```python
from build123d import *

# Parameters (mm, degrees)
BOSS_EXTRUDE1_DEPTH = 200
SKETCH2_R           = 2.5
CUT_EXTRUDE1_DEPTH  = 203.484567313


with BuildPart() as part:
    # Sketch1 → Boss-Extrude1 (new body)
    with BuildSketch(Plane.XY):
        with BuildLine():
            Line((-8.5, 10), (-3.8, 10))
            ThreePointArc((-3.8, 10), (-3.658578644, 9.941421356), (-3.6, 9.8))
            Line((-3.6, 9.8), (-3.6, 9.7))
            ThreePointArc((-3.6, 9.7), (-3.541421356, 9.558578644), (-3.4, 9.5))
            Line((-3.4, 9.5), (-3.3, 9.5))
            ThreePointArc((-3.3, 9.5), (-3.158578644, 9.441421356), (-3.1, 9.3))
            Line((-3.1, 9.3), (3.1, 9.3))
            ThreePointArc((3.1, 9.3), (3.158578644, 9.441421356), (3.3, 9.5))
            Line((3.3, 9.5), (3.4, 9.5))
            ThreePointArc((3.4, 9.5), (3.541421356, 9.558578644), (3.6, 9.7))
            Line((3.6, 9.7), (3.6, 9.8))
            ThreePointArc((3.6, 9.8), (3.658578644, 9.941421356), (3.8, 10))
            Line((3.8, 10), (8.5, 10))
            Line((8.5, 10), (11.5, 10))
            Line((11.5, 10), (16.2, 10))
            ThreePointArc((16.2, 10), (16.341421356, 9.941421356), (16.4, 9.8))
            Line((16.4, 9.8), (16.4, 9.7))
            ThreePointArc((16.4, 9.7), (16.458578644, 9.558578644), (16.6, 9.5))
            Line((16.6, 9.5), (16.7, 9.5))
            ThreePointArc((16.7, 9.5), (16.841421356, 9.441421356), (16.9, 9.3))
            Line((16.9, 9.3), (16.9, 8.2))
            Line((16.9, 8.2), (14.7, 8.2))
            ThreePointArc((14.7, 8.2), (14.558578644, 8.141421356), (14.5, 8))
            Line((14.5, 8), (14.5, 6.560660172))
            Line((14.5, 6.560660172), (17.102081528, 3.958578644))
            ThreePointArc((17.102081528, 3.958578644), (17.166966198, 3.915224093), (17.243502884, 3.9))
            Line((17.243502884, 3.9), (22.756497116, 3.9))
            ThreePointArc((22.756497116, 3.9), (22.833033802, 3.915224093), (22.897918472, 3.958578644))
            Line((22.897918472, 3.958578644), (25.5, 6.560660172))
            Line((25.5, 6.560660172), (25.5, 8))
            ThreePointArc((25.5, 8), (25.441421356, 8.141421356), (25.3, 8.2))
            Line((25.3, 8.2), (23.1, 8.2))
            Line((23.1, 8.2), (23.1, 9.3))
            ThreePointArc((23.1, 9.3), (23.158578644, 9.441421356), (23.3, 9.5))
            Line((23.3, 9.5), (23.4, 9.5))
            ThreePointArc((23.4, 9.5), (23.541421356, 9.558578644), (23.6, 9.7))
            Line((23.6, 9.7), (23.6, 9.8))
            ThreePointArc((23.6, 9.8), (23.658578644, 9.941421356), (23.8, 10))
            Line((23.8, 10), (28.5, 10))
            ThreePointArc((28.5, 10), (29.560660172, 9.560660172), (30, 8.5))
            Line((30, 8.5), (30, 3.8))
            ThreePointArc((30, 3.8), (29.941421356, 3.658578644), (29.8, 3.6))
            Line((29.8, 3.6), (29.7, 3.6))
            ThreePointArc((29.7, 3.6), (29.558578644, 3.541421356), (29.5, 3.4))
            Line((29.5, 3.4), (29.5, 3.3))
            ThreePointArc((29.5, 3.3), (29.441421356, 3.158578644), (29.3, 3.1))
            Line((29.3, 3.1), (28.2, 3.1))
            Line((28.2, 3.1), (28.2, 5.3))
            ThreePointArc((28.2, 5.3), (28.141421356, 5.441421356), (28, 5.5))
            Line((28, 5.5), (26.560660172, 5.5))
            Line((26.560660172, 5.5), (23.958578644, 2.897918472))
            ThreePointArc((23.958578644, 2.897918472), (23.915224093, 2.833033802), (23.9, 2.756497116))
            Line((23.9, 2.756497116), (23.9, -2.756497116))
            ThreePointArc((23.9, -2.756497116), (23.915224093, -2.833033802), (23.958578644, -2.897918472))
            Line((23.958578644, -2.897918472), (26.560660172, -5.5))
            Line((26.560660172, -5.5), (28, -5.5))
            ThreePointArc((28, -5.5), (28.141421356, -5.441421356), (28.2, -5.3))
            Line((28.2, -5.3), (28.2, -3.1))
            Line((28.2, -3.1), (29.3, -3.1))
            ThreePointArc((29.3, -3.1), (29.441421356, -3.158578644), (29.5, -3.3))
            Line((29.5, -3.3), (29.5, -3.4))
            ThreePointArc((29.5, -3.4), (29.558578644, -3.541421356), (29.7, -3.6))
            Line((29.7, -3.6), (29.8, -3.6))
            ThreePointArc((29.8, -3.6), (29.941421356, -3.658578644), (30, -3.8))
            Line((30, -3.8), (30, -8.5))
            ThreePointArc((30, -8.5), (29.560660172, -9.560660172), (28.5, -10))
            Line((28.5, -10), (23.8, -10))
            ThreePointArc((23.8, -10), (23.658578644, -9.941421356), (23.6, -9.8))
            Line((23.6, -9.8), (23.6, -9.7))
            ThreePointArc((23.6, -9.7), (23.541421356, -9.558578644), (23.4, -9.5))
            Line((23.4, -9.5), (23.3, -9.5))
            ThreePointArc((23.3, -9.5), (23.158578644, -9.441421356), (23.1, -9.3))
            Line((23.1, -9.3), (23.1, -8.2))
            Line((23.1, -8.2), (25.3, -8.2))
            ThreePointArc((25.3, -8.2), (25.441421356, -8.141421356), (25.5, -8))
            Line((25.5, -8), (25.5, -6.560660172))
            Line((25.5, -6.560660172), (22.897918472, -3.958578644))
            ThreePointArc((22.897918472, -3.958578644), (22.833033802, -3.915224093), (22.756497116, -3.9))
            Line((22.756497116, -3.9), (17.243502884, -3.9))
            ThreePointArc((17.243502884, -3.9), (17.166966198, -3.915224093), (17.102081528, -3.958578644))
            Line((17.102081528, -3.958578644), (14.5, -6.560660172))
            Line((14.5, -6.560660172), (14.5, -8))
            ThreePointArc((14.5, -8), (14.558578644, -8.141421356), (14.7, -8.2))
            Line((14.7, -8.2), (16.9, -8.2))
            Line((16.9, -8.2), (16.9, -9.3))
            ThreePointArc((16.9, -9.3), (16.841421356, -9.441421356), (16.7, -9.5))
            Line((16.7, -9.5), (16.6, -9.5))
            ThreePointArc((16.6, -9.5), (16.458578644, -9.558578644), (16.4, -9.7))
            Line((16.4, -9.7), (16.4, -9.8))
            ThreePointArc((16.4, -9.8), (16.341421356, -9.941421356), (16.2, -10))
            Line((16.2, -10), (11.5, -10))
            Line((11.5, -10), (8.5, -10))
            Line((8.5, -10), (3.8, -10))
            ThreePointArc((3.8, -10), (3.658578644, -9.941421356), (3.6, -9.8))
            Line((3.6, -9.8), (3.6, -9.7))
            ThreePointArc((3.6, -9.7), (3.541421356, -9.558578644), (3.4, -9.5))
            Line((3.4, -9.5), (3.3, -9.5))
            Line((3.3, -9.5), (-3.3, -9.5))
            Line((-3.3, -9.5), (-3.4, -9.5))
            ThreePointArc((-3.4, -9.5), (-3.541421356, -9.558578644), (-3.6, -9.7))
            Line((-3.6, -9.7), (-3.6, -9.8))
            ThreePointArc((-3.6, -9.8), (-3.658578644, -9.941421356), (-3.8, -10))
            Line((-3.8, -10), (-8.5, -10))
            ThreePointArc((-8.5, -10), (-9.560660172, -9.560660172), (-10, -8.5))
            Line((-10, -8.5), (-10, -3.8))
            ThreePointArc((-10, -3.8), (-9.941421356, -3.658578644), (-9.8, -3.6))
            Line((-9.8, -3.6), (-9.7, -3.6))
            ThreePointArc((-9.7, -3.6), (-9.558578644, -3.541421356), (-9.5, -3.4))
            Line((-9.5, -3.4), (-9.5, -3.3))
            ThreePointArc((-9.5, -3.3), (-9.441421356, -3.158578644), (-9.3, -3.1))
            Line((-9.3, -3.1), (-8.2, -3.1))
            Line((-8.2, -3.1), (-8.2, -5.3))
            ThreePointArc((-8.2, -5.3), (-8.141421356, -5.441421356), (-8, -5.5))
            Line((-8, -5.5), (-6.560660172, -5.5))
            Line((-6.560660172, -5.5), (-3.958578644, -2.897918472))
            ThreePointArc((-3.958578644, -2.897918472), (-3.915224093, -2.833033802), (-3.9, -2.756497116))
            Line((-3.9, -2.756497116), (-3.9, 2.756497116))
            ThreePointArc((-3.9, 2.756497116), (-3.915224093, 2.833033802), (-3.958578644, 2.897918472))
            Line((-3.958578644, 2.897918472), (-6.560660172, 5.5))
            Line((-6.560660172, 5.5), (-8, 5.5))
            ThreePointArc((-8, 5.5), (-8.141421356, 5.441421356), (-8.2, 5.3))
            Line((-8.2, 5.3), (-8.2, 3.1))
            Line((-8.2, 3.1), (-9.3, 3.1))
            ThreePointArc((-9.3, 3.1), (-9.441421356, 3.158578644), (-9.5, 3.3))
            Line((-9.5, 3.3), (-9.5, 3.4))
            ThreePointArc((-9.5, 3.4), (-9.558578644, 3.541421356), (-9.7, 3.6))
            Line((-9.7, 3.6), (-9.8, 3.6))
            ThreePointArc((-9.8, 3.6), (-9.941421356, 3.658578644), (-10, 3.8))
            Line((-10, 3.8), (-10, 8.5))
            ThreePointArc((-10, 8.5), (-9.560660172, 9.560660172), (-8.5, 10))
        make_face()
        with BuildLine():
            Line((3.9, 2.756497116), (3.9, -2.756497116))
            ThreePointArc((3.9, -2.756497116), (3.915224093, -2.833033802), (3.958578644, -2.897918472))
            Line((3.958578644, -2.897918472), (6.560660172, -5.5))
            Line((6.560660172, -5.5), (6.560660172, -8.2))
            Line((6.560660172, -8.2), (13.439339828, -8.2))
            Line((13.439339828, -8.2), (13.439339828, -5.5))
            Line((13.439339828, -5.5), (16.041421356, -2.897918472))
            ThreePointArc((16.041421356, -2.897918472), (16.084775907, -2.833033802), (16.1, -2.756497116))
            Line((16.1, -2.756497116), (16.1, 2.756497116))
            ThreePointArc((16.1, 2.756497116), (16.084775907, 2.833033802), (16.041421356, 2.897918472))
            Line((16.041421356, 2.897918472), (13.439339828, 5.5))
            Line((13.439339828, 5.5), (13.439339828, 8.2))
            Line((13.439339828, 8.2), (6.560660172, 8.2))
            Line((6.560660172, 8.2), (6.560660172, 5.5))
            Line((6.560660172, 5.5), (3.958578644, 2.897918472))
            ThreePointArc((3.958578644, 2.897918472), (3.915224093, 2.833033802), (3.9, 2.756497116))
        make_face(mode=Mode.SUBTRACT)
    extrude(amount=BOSS_EXTRUDE1_DEPTH)

    # Sketch2 → Cut-Extrude1 (cut, through all)
    with BuildSketch(Plane.XY.offset(200)):
        Circle(SKETCH2_R)
        with Locations(Location((20, 0, 0), (0, 0, 180))):
            Circle(SKETCH2_R)
    extrude(amount=-CUT_EXTRUDE1_DEPTH, mode=Mode.SUBTRACT)


solid = part.part
```
Geometry check sheet. Reference: the model listing, model coordinates, mm. A direction names the side the tool comes from. Coordinates: 2 decimals unless noted, no trailing zeros. Order: outer loops, then holes, each group sorted by start corner. A loop starts at its lowest first (then second) coordinate and runs counter-clockwise, first axis right, second up.
Item 1: Scan lines: line 1 along X through (y, z) = (-7.25, 171); line 2 along Y through (x, z) = (0, 93); line 3 along X through (y, z) = (2.25, 39.5). Record each from-to range of solid material in increasing order.
Item 2: Mould release check, pull along Y, two halves, no side actions. Record for faces 4 (the flat face through (10, 10, 99)), 5 (the flat face through (10, -8.2, 99)), 6 (the flat face through (6, 7, 200)): released by +Y, released by -Y, zero draft, split by the parting line, or undercut.
Item 3: Section check A-A (y = 0). Enter the section's corners in (x, z).
Item 4: Tool access check on faces 1 (the flat face through (23.9, 0, 99)), 2 (the flat face through (0, -9.5, 99)), 3 (the flat face through (20, 3.9, 99)). Record the directions out of +Z, -Z, +X, -X, +Y, -Y that give a thin tool (end or side, any length) a straight path to the whole face; none if there is none.
Item 5: Section check C-C (x = 0). Enter the section's corners in (y, z), plus the area to 3 significant figures.
Item 6: Section check B-B (x = 20). Enter the section's corners in (y, z), plus the area to 3 significant figures.
Item 7: Section check D-D (z = 54.5). Count the separate pieces of the cut face and the enclosed holes in it, plus the area to 3 significant figures.
Item 8: Depth check by flat-ended pin: pin 1 (3 mm diameter, centred on y = 0.5, z = 87, fed in from +X); pin 2 (4.5 mm diameter, centred on y = -0.5, z = 76, fed in from -X). Enter the tip coordinate at first touch or a pass-through.
Check sheet entries:
1. line 1: x = -10 to 6.56, 13.44 to 14.5, 25.5 to 30
1. line 2: y = -9.5 to -2.5, 2.5 to 9.3
1. line 3: x = -3.9 to -1.09, 1.09 to 3.9, 16.1 to 18.91, 21.09 to 23.9
2. face 4: released by +Y
2. face 5: undercut
2. face 6: zero draft
3. outline: (-3.9, 0) - (-2.5, 0) - (-2.5, 200) - (-3.9, 200) - close; (2.5, 0) - (3.9, 0) - (3.9, 200) - (2.5, 200) - close; (16.1, 0) - (17.5, 0) - (17.5, 200) - (16.1, 200) - close; (22.5, 0) - (23.9, 0) - (23.9, 200) - (22.5, 200) - close
4. face 1: +Z, -Z, +X
4. face 2: +Z, -Z, -Y
4. face 3: +Z, -Z, +Y
5. outline: (-9.5, 0) - (-2.5, 0) - (-2.5, 200) - (-9.5, 200) - close; (2.5, 0) - (9.3, 0) - (9.3, 200) - (2.5, 200) - close
5. area: 2,760 mm2
6. outline: (-3.9, 0) - (-2.5, 0) - (-2.5, 200) - (-3.9, 200) - close; (2.5, 0) - (3.9, 0) - (3.9, 200) - (2.5, 200) - close
6. area: 560 mm2
7. separate pieces: 1
7. enclosed holes: 3
7. area: 386 mm2
8. pin 1: stops at x = 23.9
8. pin 2: stops at x = -3.9
